Answer from the drawing. Dimensions are ordinates in mm from the lowest x, y and z of the part. Give positions to 0.01 mm unless a question says otherwise; leave off trailing zeros. Loops run counter-clockwise (first coordinate to the right, second up) from the corner with the lowest first, then second, coordinate; pieces in that order, holes last. Notation, with made-up numbers: (7, 53.5) - (59, 53.5) arc R16 ccw to (59, 81.5) - close; hole circle Ø6 at (-36.5, 42.5). An arc over 180 degrees is marked (long way). Write each question's results on one line, items separated by ' | '. Start each with the question number.
Q1. The part is cut by section A-A, the plane x = 7.5. Write down the section's boundary in (y, z), plus the area to 3 significant figures.
Q2. Find the intervals of material crossed by line 1 (X direction, y = 4.25, z = 7.5); line 2 (Z direction, x = 6.5, y = 2.5); line 3 (Z direction, x = 5, y = 9), in increasing order. Write a range as from..to.
Q3. The part is cut by section B-B, the plane z = 7.5. Write down the section's boundary in (x, y), plus the area to 3 significant figures.
Q4. Determine the mould class of the marked faces 1, 2, 3 and 4 for opening direction X: +X half, -X half, draft (parallel to the pull), parting line (faces both ways), or undercut.
Q5. The part is cut by section C-C, the plane y = 8. Write down the section's boundary in (x, z).
Q6. The part is cut by section D-D, the plane y = 10. Write down the section's boundary in (x, z).
Q7. Given pin 1 (2 mm diameter, centred on x = 10.5, y = 3.5, fed in from -Z); pin 2 (6 mm diameter, centred on y = 1.5, z = 12.5, fed in from +X); pin 3 (4 mm diameter, centred on x = 7.5, z = 7.5, fed in from -Y); pin 4 (1 mm diameter, centred on y = 10, z = 2.5, fed in from -X), each flat-ended and moving along its own axis, determine where each tip first touches the part or whether it passes through.
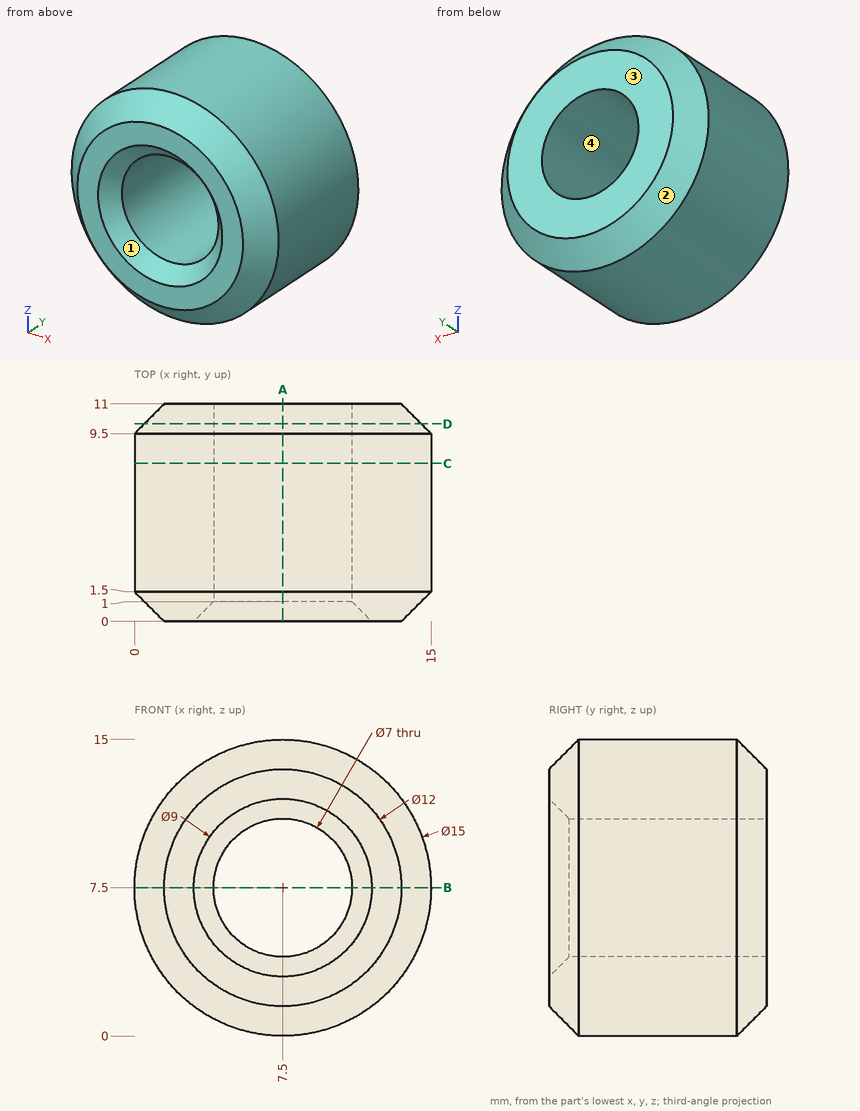
Check sheet entries:
1) outline: (0, 1.5) - (1.5, 0) - (9.5, 0) - (11, 1.5) - (11, 4) - (1, 4) - (0, 3) - close; (0, 12) - (1, 11) - (11, 11) - (11, 13.5) - (9.5, 15) - (1.5, 15) - (0, 13.5) - close | area: 82.5 mm^2
2) line 1: x = 0..4, 11..15 | line 2: z = 0.07..4.15, 10.85..14.93 | line 3: z = 0.43..5.05, 9.95..14.57
3) outline: (0, 1.5) - (1.5, 0) - (3, 0) - (4, 1) - (4, 11) - (1.5, 11) - (0, 9.5) - close; (11, 1) - (12, 0) - (13.5, 0) - (15, 1.5) - (15, 9.5) - (13.5, 11) - (11, 11) - close | area: 82.5 mm^2
4) face 1: undercut | face 2: parting line | face 3: draft | face 4: undercut
5) outline: circle Ø15 at (7.5, 7.5); hole circle Ø7 at (7.5, 7.5)
6) outline: circle Ø14 at (7.5, 7.5); hole circle Ø7 at (7.5, 7.5)
7) pin 1: stops at z = 0.27 | pin 2: stops at x = 14.73 | pin 3: passes through | pin 4: stops at x = 1.78
